Source: CAD feature listing. Evaluate the final solid. Frame: model axes, mm. A direction names the side the tool comes from. Give positions to 0.01 mm unless a question says otherwise; leave off trailing zeros. Order: outer loops, then holes, each group sorted by start corner. A loop starts at its lowest first (then second) coordinate and runs counter-clockwise, first axis right, second up.
```python
from build123d import *

# Parameters (mm, degrees)
SKETCH_1_R          = 3
EXTRUDE_1_DEPTH     = 0.8
CUT_EXTRUDE_1_DEPTH = 0.5


# Read off the part's stored shape, not the designer's step: M3 机械螺纹 螺柱3
with BuildPart() as part:
    # 草图1 → 凸台-拉伸1 (new body)
    with BuildSketch(Plane(origin=(0, 0, 0), x_dir=(1, 0, 0), z_dir=(0, 1, 0))):
        with Locations(Location((0, 0, 0), (0, 0, 270))):
            Circle(SKETCH_1_R)
    extrude(amount=EXTRUDE_1_DEPTH)

    # M3 机械螺纹 螺柱3 outline → M3 机械螺纹 螺柱3 (revolve)
    with BuildSketch(Plane.XY):
        Polygon((1.2295, 6.8), (0, 6.8), (0, 0.8), (1.5, 0.8), (1.5, 6.5295), align=None)
    revolve(axis=Axis((0, 0, 0), (0, 1, 0)))

    # 草图8 → 切除-拉伸1 (cut)
    with BuildSketch(Plane.XZ):
        Polygon((1.154700538, 0), (0.577350269, 1), (-0.577350269, 1), (-1.154700538, 0), (-0.577350269, -1), (0.577350269, -1), align=None)
    extrude(amount=-CUT_EXTRUDE_1_DEPTH, mode=Mode.SUBTRACT)


solid = part.part
```
1) Reachability of faces 4 (the flat face through (-1.3, 0.8, 1.3)), 5 (the flat face through (0, 6.8, 0)) from +Z, -Z, +X, -X, +Y, -Y: full face, straight path, thin tool, end or side. Return the list, or none.
Report:
face 4: +Y
face 5: +Z, -Z, +X, -X, +Y
2) Section query B-B, the plane z = -2.15. Return the cut outline in (x, y).
Report:
outline: (-2.09, 0) - (2.09, 0) - (2.09, 0.8) - (-2.09, 0.8) - close
3) Section query D-D, the plane x = 2.4. Return the cut outline in (y, z).
Report:
outline: (0, -1.8) - (0.8, -1.8) - (0.8, 1.8) - (0, 1.8) - close
4) Section query A-A, the plane x = 0. Return the cut outline in (y, z).
Report:
outline: (0, -3) - (0.8, -3) - (0.8, -1.5) - (6.53, -1.5) - (6.8, -1.23) - (6.8, 1.23) - (6.53, 1.5) - (0.8, 1.5) - (0.8, 3) - (0, 3) - (0, 1) - (0.5, 1) - (0.5, -1) - (0, -1) - close
5) Draft query along X for faces 1 (the cylindrical face through (0.9, 0.39, 2.86)), 2 (the flat face through (0, 0.5, 0)), 3 (the flat face through (0, 0, 1.3)). Return one class per face: +X half, -X half, draft (parallel to the pull), parting line (faces both ways), or undercut.
Report:
face 1: parting line
face 2: undercut
face 3: draft
6) Material intervals for L1, parallel to Y at x = 2.2, z = -0.45; L2, parallel to Z at x = -0.85, y = 1.25; L3, parallel to Z at x = 0.3, y = 5.5, sorted ascending.
Report:
L1: y = 0 to 0.8
L2: z = -1.24 to 1.24
L3: z = -1.47 to 1.47
7) Pin query (flat end, axial travel): pin 1 (2 mm diameter, centred on x = -1.5, y = 6, fed in from -Z); pin 2 (1 mm diameter, centred on y = 3.5, z = -1.5, fed in from +X); pin 3 (1.6 mm diameter, centred on x = 0, z = 0, fed in from -Y). Return the tip coordinate at first contact, or that it passes through.
Report:
pin 1: stops at z = -1.41
pin 2: stops at x = 1.12
pin 3: stops at y = 0.5
8) Section query C-C, the plane y = 6. Return the cut outline in (x, z).
Report:
outline: circle Ø3 at (0, 0)
